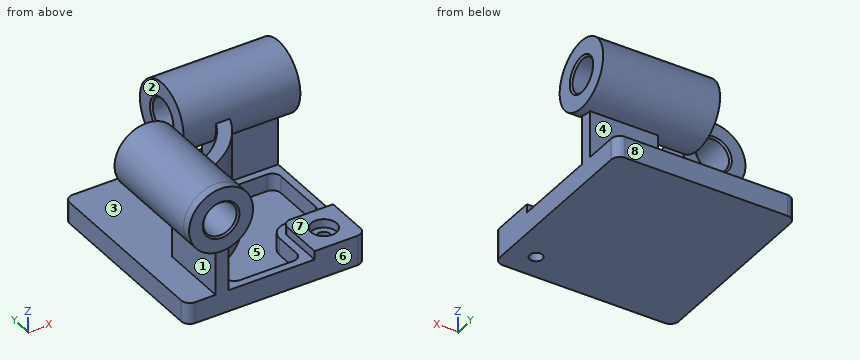
```python
from build123d import *

# Parameters (mm, degrees)
F0_W            = 210
F0_H            = 225
F1_DEPTH        = 25
F3_DEPTH        = 95
F4_R            = 37.5
F5_DEPTH        = 10
F5_DEPTH_BACK   = 127
F6_R            = 40
F7_DEPTH        = 10
F7_DEPTH_BACK   = 127
F8_W            = 60
F8_H            = 60
F9_DEPTH        = 10
F10_R           = 10
F12_DEPTH       = 20
F14_D           = 15
F14_CBORE_D     = 30
F14_CBORE_DEPTH = 10
F15_R           = 10
F16_R           = 19.5
F17_DEPTH       = 235.001
F18_R           = 19.5
F19_DEPTH       = 223.501
F20_SIZE        = 2
F21_R           = 10


with BuildPart() as f1:
    # F0 (on Top) → F1 (new body)
    with BuildSketch(Plane.XY):
        Rectangle(F0_W, F0_H)
    extrude(amount=F1_DEPTH)

    # F2 (on face) → F3 (join)
    with BuildSketch(Plane.XY.offset(25)):
        with BuildLine():
            Line((-71, -32.5), (-71, -112.5))
            Line((-71, -112.5), (-56.000001, -112.5))
            Line((-56.000001, -112.5), (-56.000001, -46.481815))
            ThreePointArc((-56.000001, -46.481815), (7.488852, -14.988852), (38.981815, 48.500001))
            Line((38.981815, 48.500001), (105, 48.500001))
            Line((105, 48.500001), (105, 63.5))
            Line((105, 63.5), (25, 63.5))
            ThreePointArc((25, 63.5), (-3.117749, -4.382251), (-71, -32.5))
        make_face()
    extrude(amount=F3_DEPTH)

    # F4 (on face) → F5 (join, two sides)
    with BuildSketch(Plane.XZ.offset(112.5)) as f5_sk:
        with Locations((-71, 120)):
            Circle(F4_R)
    extrude(amount=F5_DEPTH)
    extrude(f5_sk.sketch, amount=-F5_DEPTH_BACK)

    # F6 (on face) → F7 (join, two sides)
    with BuildSketch(Plane.YZ.offset(105)) as f7_sk:
        with Locations((63.5, 120)):
            Circle(F6_R)
    extrude(amount=F7_DEPTH)
    extrude(f7_sk.sketch, amount=-F7_DEPTH_BACK)

    # F8 (on face) → F9 (join)
    with BuildSketch(Plane.XY.offset(25)):
        with Locations((75, -82.5)):
            Rectangle(F8_W, F8_H)
    extrude(amount=F9_DEPTH)

    # F10
    f10_edges = [f1.edges().sort_by_distance(p)[0] for p in [
        (45, -52.5, 30),
    ]]
    fillet(f10_edges, radius=F10_R)

    # F11 (on face) → F12 (cut)
    with BuildSketch(Plane.XY.offset(25)):
        with BuildLine():
            ThreePointArc((46.575506, 39.500001), (13.852813, -21.352813), (-47.000001, -54.075506))
            Line((-47.000001, -54.075506), (-47.000001, -103.5))
            Line((-47.000001, -103.5), (36, -103.5))
            Line((36, -103.5), (36, -62.5))
            ThreePointArc((36, -62.5), (41.564971, -49.064971), (55, -43.5))
            Line((55, -43.5), (96, -43.5))
            Line((96, -43.5), (96, 39.500001))
            Line((96, 39.500001), (46.575506, 39.500001))
        make_face()
    extrude(amount=-F12_DEPTH, mode=Mode.SUBTRACT)

    # F14 (through all)
    with Locations(Plane.XY.offset(35)):
        with Locations((75, -82.5)):
            CounterBoreHole(F14_D / 2, F14_CBORE_D / 2, F14_CBORE_DEPTH)

    # F15
    f15_edges = [f1.edges().sort_by_distance(p)[0] for p in [
        (-47.000001, -54.075506, 15),
        (46.575506, 39.500001, 15),
        (96, 39.500001, 15),
        (-47.000001, -103.5, 15),
        (36, -103.5, 15),
        (96, -43.5, 15),
    ]]
    fillet(f15_edges, radius=F15_R)

    # F16 (on face) → F17 (cut, through all)
    with BuildSketch(Plane.XZ.offset(122.5)):
        with Locations((-71, 120)):
            Circle(F16_R)
    extrude(amount=-F17_DEPTH, mode=Mode.SUBTRACT)

    # F18 (on face) → F19 (cut, through all)
    with BuildSketch(Plane.YZ.offset(115)):
        with Locations((63.5, 120)):
            Circle(F18_R)
    extrude(amount=-F19_DEPTH, mode=Mode.SUBTRACT)

    # F20
    f20_edges = [f1.edges().sort_by_distance(p)[0] for p in [
        (-90.5, -122.5, 120),
        (115, 44, 120),
        (-22, 44, 120),
        (-90.5, 14.5, 120),
    ]]
    chamfer(f20_edges, length=F20_SIZE)

    # F21
    f21_edges = [f1.edges().sort_by_distance(p)[0] for p in [
        (105, -112.5, 17.5),
        (105, 112.5, 12.5),
        (-105, -112.5, 12.5),
        (-105, 112.5, 12.5),
    ]]
    fillet(f21_edges, radius=F21_R)


solid = f1.part
```
Part model, mm, in its own coordinate system. Face numbers are marked on the shaded views. A direction names the side the tool comes from. Give positions to 0.01 mm unless a question says otherwise; leave off trailing zeros. Order: outer loops, then holes, each group sorted by start corner. A loop starts at its lowest first (then second) coordinate and runs counter-clockwise, first axis right, second up. Notation, with made-up numbers: (8.5, -19.75) - (43.5, -19.75) arc R16 ccw to (43.5, 5.25) - close; hole circle Ø6 at (63.25, 84). An arc over 180 degrees is marked (long way). Use one line per item in the form item = value.
Item 1: Slice it at B-B on y = -82.5. Give the cut face in (x, z).
Solution:
outline = (-105, 0) - (67.5, 0) - (67.5, 25) - (60, 25) - (60, 35) - (45, 35) - (45, 25) - (36, 25) - (36, 5) - (-47, 5) - (-47, 25) - (-56, 25) - (-56, 85.63) arc R37.5 ccw (long way) to (-71, 82.5) - (-71, 25) - (-105, 25) - close; (82.5, 0) - (105, 0) - (105, 35) - (90, 35) - (90, 25) - (82.5, 25) - close; hole circle Ø39 at (-71, 120)
Item 2: Slice it at A-A on x = 75. Give the cut face in (y, z).
Solution:
outline = (-112.5, 0) - (-90, 0) - (-90, 25) - (-97.5, 25) - (-97.5, 35) - (-112.5, 35) - close; (-75, 0) - (112.5, 0) - (112.5, 25) - (63.5, 25) - (63.5, 80) arc R40 ccw (long way) to (48.5, 82.92) - (48.5, 25) - (39.5, 25) - (39.5, 5) - (-43.5, 5) - (-43.5, 25) - (-52.5, 25) - (-52.5, 35) - (-67.5, 35) - (-67.5, 25) - (-75, 25) - close; hole circle Ø39 at (63.5, 120)
Item 3: Two-plate mould, pull along Y, no slides. Class the marked faces 5, 6, 7 and 8: released by +Y, released by -Y, zero draft, split by the parting line, or undercut.
Solution:
face_5 = undercut
face_6 = released by -Y
face_7 = zero draft
face_8 = released by +Y
Item 4: Pin check, flat tips, straight feed: pin 1 Ø10 at (y, z) = (36, 34) entering from -X; pin 2 Ø18 at (x, y) = (66, -86) entering from +Z; pin 3 Ø1.5 at (x, z) = (46, 87.5) entering from -Y; pin 4 Ø10 at (x, y) = (-32, 12.5) entering from -Z. Stop position of each tip, or through.
Solution:
pin_1 = 19.33
pin_2 = 35
pin_3 = 39.17
pin_4 = 0
Item 5: Which spindle directions (+Z, -Z, +X, -X, +Y, -Y) get a long thin tool onto all of the face, cutting with end or side? Do the marked faces 1, 2, 3 and 4. Say none if no direction does.
Solution:
face_1 = -X, +Y, -Y
face_2 = +Z, -X, +Y
face_3 = -X, +Y
face_4 = +X, -X, +Y
Item 6: Probe probe 1 along Z at (x, y) = (-71, -16); probe 2 along Y at (x, z) = (75, 13.5); probe 3 along Y at (x, z) = (53, 118.5). List the from-to ranges inside material, lowest first. Write a range as from..to.
Solution:
probe_1 = 0..25, 82.5..100.5, 139.5..157.5
probe_2 = -112.5..-90, -75..-43.5, 39.5..112.5
probe_3 = 23.53..44.06, 82.94..103.47
